Could you check a few things on this model? Use its own coordinates, in mm. A direction names the side the tool comes from. Round coordinates to 2 decimals unless told otherwise and drop trailing zeros. Write each loop counter-clockwise with the first axis right and the second up, starting at its lowest first coordinate (ties: lowest second). Pieces come first, ordered by that corner, then holes. Notation, with made-up numbers: (-18.5, 0.5) - (-8.5, 0.5) arc R28 ccw to (-8.5, 33.5) - close; hole circle Ø3 at (34, 67). An arc over 180 degrees is marked (long way). Write each question's results on one line, items separated by ' | '. Start each with the question number.
(1) Please list where these lines run through material, in increasing order: line 1 (X direction, y = 396, z = -25); line 2 (Z direction, x = 178.5, y = 128); line 3 (X direction, y = 346.5, z = -5.5). Write a range as [from, to].
(2) Imagine slicing it at D-D on x = 154. Write out the boundary of the cut face in (y, z).
(3) Imagine slicing it at B-B on y = 284.5. Write out the boundary of the cut face in (x, z), then the cut area to 3 significant figures.
(4) Thinking about a two-plate mould opening in X: for faces 1 (the cylindrical face through (191.41, 234.18, -4.26)), 2 (the cylindrical face through (-191.59, 234.18, -4.44)), 3 (the cylindrical face through (-192.03, 234.18, -3.62)), 4 (the flat face through (-191.4, 475, -4)), which applies, +X half, -X half, draft (parallel to the pull), parting line (faces both ways), or undercut?
(5) Imagine slicing it at C-C on x = -51. Write out the boundary of the cut face in (y, z), then the cut area to 3 significant figures.
(6) On a 3-axis mill with a long thin cutter (end or side, diameter ignored), from which of +Z, -Z, +X, -X, +Y, -Y can I reach the whole of each face in a straight line? I mean faces 5 (the flat face through (192, 475, -4)), 6 (the flat face through (3, 340, 0)), 7 (the flat face through (194.961, 234, -38)). Say none if no direction works.
(7) For P1, Ø8, axis at x = 138, z = -11, coming from the -Y side; P2, Ø7, axis at y = 30, z = -50.1, coming from the -X side; P3, Ø7, axis at x = -118.95, y = 316.13, coming from the -Z side; P4, Ø4, axis at y = 60, z = -50.1, coming from the +X side, each with a flat end and sliding along its axis, tell me the tip position at first contact or that it passes through.
(8) Imagine slicing it at A-A on x = 11. Write out the boundary of the cut face in (y, z), then the cut area to 3 significant figures.
```python
from build123d import *

# Parameters (mm, degrees)
BASE_FLANGE2_DEPTH        = 475
SKETCH6_W                 = 225
SKETCH6_H                 = 225
CUT_EXTRUDE2_DEPTH        = 2.54
SKETCH13_R                = 2.25
CUT_EXTRUDE4_DEPTH        = 619.939427238
SKETCH14_R                = 2.25
CUT_EXTRUDE5_DEPTH        = 0.889
SKETCH15_W                = 70
SKETCH15_H                = 20
CUT_EXTRUDE6_DEPTH        = 0.889
EDGE_FLANGE1_DEPTH        = 50.8
EDGE_FLANGE1_BEND_DEPTH   = 366.299839916
EDGE_FLANGE1_BEND_2_DEPTH = 50.8
BREAK_CORNER1_START       = 475.381
BREAK_CORNER1_DEPTH       = 0.889


# Read off the part's stored shape, not the designer's step: Break-Corner1
# Sheet-metal steps are written as plain solids
with BuildPart() as part:
    # Sketch1 → Base-Flange2 (new body)
    with BuildSketch(Plane(origin=(0, 0, 0), x_dir=(1, 0, 0), z_dir=(0, 1, 0))):
        with BuildLine():
            Line((195.849919958, 63.5), (195.849919958, 12.7))
            ThreePointArc((195.849919958, 12.7), (192.130176079, 3.719743879), (183.149919958, 0))
            Line((183.149919958, 0), (-183.149919958, 0))
            ThreePointArc((-183.149919958, 0), (-192.130176079, 3.719743879), (-195.849919958, 12.7))
            Line((-195.849919958, 12.7), (-195.849919958, 63.5))
            Line((-195.849919958, 63.5), (-194.960919958, 63.5))
            Line((-194.960919958, 63.5), (-194.960919958, 12.7))
            ThreePointArc((-194.960919958, 12.7), (-191.501558151, 4.348361807), (-183.149919958, 0.889))
            Line((-183.149919958, 0.889), (183.149919958, 0.889))
            ThreePointArc((183.149919958, 0.889), (191.501558151, 4.348361807), (194.960919958, 12.7))
            Line((194.960919958, 12.7), (194.960919958, 63.5))
            Line((194.960919958, 63.5), (195.849919958, 63.5))
        make_face()
    extrude(amount=BASE_FLANGE2_DEPTH)

    # Sketch6 → Cut-Extrude2 (cut)
    with BuildSketch(Plane.XY):
        with Locations((0, 187.5)):
            Rectangle(SKETCH6_W, SKETCH6_H)
    extrude(amount=-CUT_EXTRUDE2_DEPTH, mode=Mode.SUBTRACT)

    # Sketch13 → Cut-Extrude4 (cut, through all)
    with BuildSketch(Plane(origin=(195.849919958, 0, 0), x_dir=(0, 0, -1), z_dir=(1, 0, 0))):
        with Locations((50.096107, 60)):
            Circle(SKETCH13_R)
        with Locations((50.096107, 316.132840032)):
            Circle(SKETCH13_R)
        with Locations((50.096107, 30)):
            Circle(SKETCH13_R)
    extrude(amount=-CUT_EXTRUDE4_DEPTH, mode=Mode.SUBTRACT)

    # Sketch14 → Cut-Extrude5 (cut)
    with BuildSketch(Plane.XY):
        with Locations((-145.753813013, 316.132839976)):
            Circle(SKETCH14_R)
        with Locations((-118.946026903, 316.132839976)):
            Circle(SKETCH14_R)
        with Locations((118.946026903, 316.132839976)):
            Circle(SKETCH14_R)
        with Locations((145.753813013, 316.132839976)):
            Circle(SKETCH14_R)
        with Locations((145.753813013, 59.61392)):
            Circle(SKETCH14_R)
        with Locations((118.946026903, 59.61392)):
            Circle(SKETCH14_R)
        with Locations((-118.946026903, 59.61392)):
            Circle(SKETCH14_R)
        with Locations((-145.753813013, 59.61392)):
            Circle(SKETCH14_R)
    extrude(amount=-CUT_EXTRUDE5_DEPTH, mode=Mode.SUBTRACT)

    # Sketch15 → Cut-Extrude6 (cut)
    with BuildSketch(Plane.XY):
        with Locations((-50, 22)):
            Rectangle(SKETCH15_W, SKETCH15_H)
    extrude(amount=-CUT_EXTRUDE6_DEPTH, mode=Mode.SUBTRACT)

    # Edge-Flange1 section (across the edge) → Edge-Flange1 (add)
    with BuildSketch(Plane(origin=(-194.960919958, 475.381, -63.5), x_dir=(0, -1, 0), z_dir=(0, 0, 1))):
        with BuildLine():
            Line((-0.889, 0.381), (-0.889, 9.111))
            Line((-0.889, 9.111), (0, 9.111))
            Line((0, 9.111), (0, 0.381))
            ThreePointArc((0, 0.381), (0.111592316, 0.111592316), (0.381, 0))
            Line((0.381, 0), (0.381, -0.889))
            ThreePointArc((0.381, -0.889), (-0.517025612, -0.517025612), (-0.889, 0.381))
        make_face()
    extrude(amount=EDGE_FLANGE1_DEPTH)

    # Edge-Flange1 section 2 (across the edge) → Edge-Flange1 bend (add)
    with BuildSketch(Plane(origin=(-183.149919958, 475.381, -0.889), x_dir=(0, -1, 0), z_dir=(1, 0, 0))):
        with BuildLine():
            Line((-0.889, 0.381), (-0.889, 9.111))
            Line((-0.889, 9.111), (0, 9.111))
            Line((0, 9.111), (0, 0.381))
            ThreePointArc((0, 0.381), (0.111592316, 0.111592316), (0.381, 0))
            Line((0.381, 0), (0.381, -0.889))
            ThreePointArc((0.381, -0.889), (-0.517025612, -0.517025612), (-0.889, 0.381))
        make_face()
    extrude(amount=EDGE_FLANGE1_BEND_DEPTH)

    # Edge-Flange1 section 3 (across the edge) → Edge-Flange1 bend 2 (add)
    with BuildSketch(Plane(origin=(194.960919958, 475.381, -12.7), x_dir=(0, -1, 0), z_dir=(0, 0, -1))):
        with BuildLine():
            Line((-0.889, 0.381), (-0.889, 9.111))
            Line((-0.889, 9.111), (0, 9.111))
            Line((0, 9.111), (0, 0.381))
            ThreePointArc((0, 0.381), (0.111592316, 0.111592316), (0.381, 0))
            Line((0.381, 0), (0.381, -0.889))
            ThreePointArc((0.381, -0.889), (-0.517025612, -0.517025612), (-0.889, 0.381))
        make_face()
    extrude(amount=EDGE_FLANGE1_BEND_2_DEPTH)

    # Break-Corner1 outline → Break-Corner1 (cut)
    with BuildSketch(Plane(origin=(0, 0, 0), x_dir=(1, 0, 0), z_dir=(0, 1, 0)).offset(BREAK_CORNER1_START)):
        Polygon((183.149919958, 10), (178.149919958, 10), (183.149919958, 5), align=None)
        Polygon((-183.149919958, 5), (-178.149919958, 10), (-183.149919958, 10), align=None)
        Polygon((185.849919958, 63.5), (185.849919958, 58.5), (190.849919958, 63.5), align=None)
        Polygon((190.849919958, 12.7), (185.849919958, 17.7), (185.849919958, 12.7), align=None)
        Polygon((-185.849919958, 12.7), (-185.849919958, 17.7), (-190.849919958, 12.7), align=None)
        Polygon((-190.849919958, 63.5), (-185.849919958, 58.5), (-185.849919958, 63.5), align=None)
    extrude(amount=BREAK_CORNER1_DEPTH, mode=Mode.SUBTRACT)


solid = part.part
```
Response:
1) line 1: [-195.85, -194.96], [194.96, 195.85] | line 2: [-0.89, 0] | line 3: [-193.61, -192.51], [192.51, 193.61]
2) outline: (0, -0.89) - (475, -0.89) arc R0.38 cw to (475.38, -1.27) - (475.38, -10) - (476.27, -10) - (476.27, -1.27) arc R1.27 ccw to (475, 0) - (0, 0) - close
3) outline: (-195.85, -63.5) - (-194.96, -63.5) - (-194.96, -12.7) arc R11.81 cw to (-183.15, -0.89) - (-112.5, -0.89) - (-112.5, 0) - (-183.15, 0) arc R12.7 ccw to (-195.85, -12.7) - close; (112.5, -0.89) - (183.15, -0.89) arc R11.81 cw to (194.96, -12.7) - (194.96, -63.5) - (195.85, -63.5) - (195.85, -12.7) arc R12.7 ccw to (183.15, 0) - (112.5, 0) - close | area: 250 mm²
4) face 1: undercut | face 2: undercut | face 3: -X half | face 4: draft
5) outline: (0, -0.89) - (12, -0.89) - (12, 0) - (0, 0) - close; (32, -0.89) - (75, -0.89) - (75, 0) - (32, 0) - close; (300, -0.89) - (475, -0.89) arc R0.38 cw to (475.38, -1.27) - (475.38, -10) - (476.27, -10) - (476.27, -1.27) arc R1.27 ccw to (475, 0) - (300, 0) - close | area: 213 mm²
6) face 5: +Z, +X, +Y | face 6: +Z, +X, -X, +Y, -Y | face 7: -Z, -Y
7) P1: y = 475.38 | P2: x = -195.85 | P3: z = -0.89 | P4: through
8) outline: (0, -0.89) - (75, -0.89) - (75, 0) - (0, 0) - close; (300, -0.89) - (475, -0.89) arc R0.38 cw to (475.38, -1.27) - (475.38, -10) - (476.27, -10) - (476.27, -1.27) arc R1.27 ccw to (475, 0) - (300, 0) - close | area: 231 mm²
